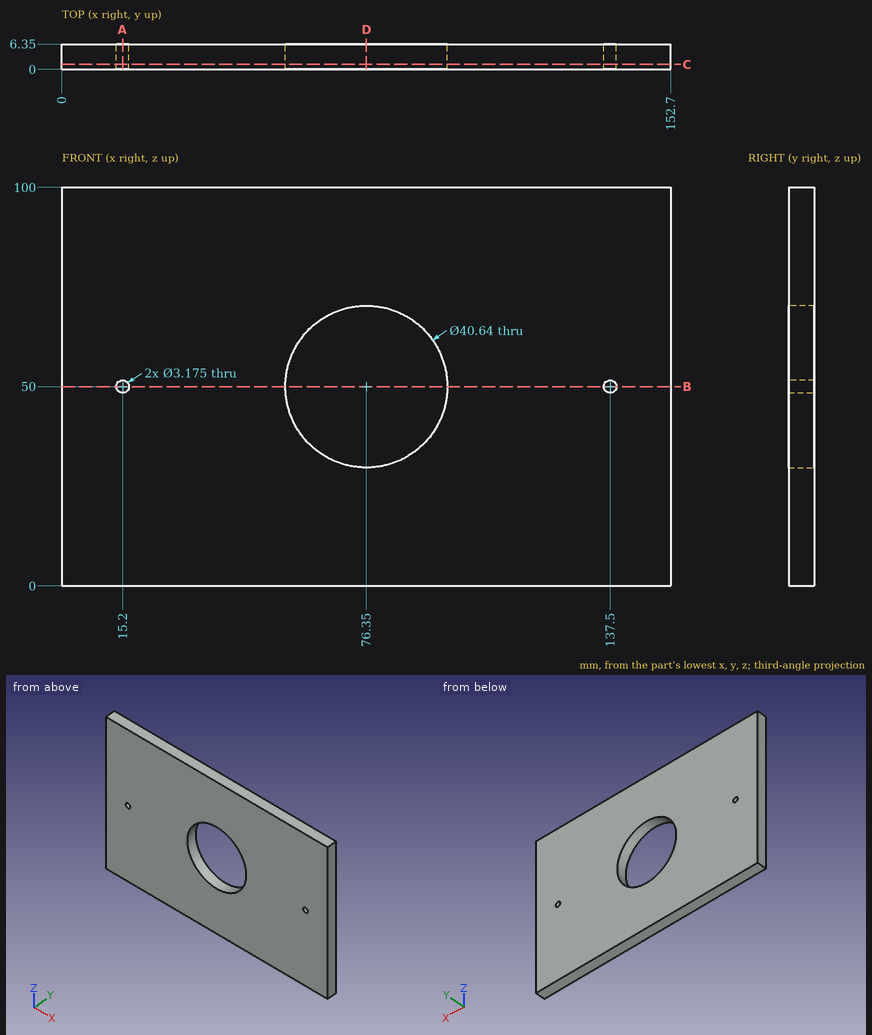
Design review of the part shown in the three views and the two pictorial views. Dimensions are in mm from the part's minimum x, y and z. Give positions to 0.01 mm unless a question says otherwise; leave off trailing zeros. Loops run counter-clockwise (first coordinate to the right, second up) from the corner with the lowest first, then second, coordinate; pieces in that order, holes last. Notation, with made-up numbers: (12, -29) - (69, -29) arc R29 ccw to (69, -4) - close; hole circle Ø3 at (86.5, -4). An arc over 180 degrees is marked (long way). Use CSV: the item, a comma, the result in double quotes. Start each with the question number.
1. Add section C-C (y = 1.25). Count the separate pieces of the cut face and the enclosed holes in it, plus the area to 3 significant figures.
2. Add section B-B (z = 50). State the section outline as (x, y) points.
3. Wall thickness on L1, parallel to X at y = 4, z = 50; L2, parallel to Z at x = 137.5, y = 4.75; L3, parallel to X at y = 2, z = 47: over which ranges is each line inside the solid? List them lowest first.
4. Add section D-D (x = 76.35). State the section outline as (y, z) points, plus the area to 3 significant figures.
5. Add section A-A (x = 15.2). State the section outline as (y, z) points, plus the area to 3 significant figures.
Results found:
1,separate pieces,"1"
1,enclosed holes,"3"
1,area,"14,000 mm²"
2,outline,"(0, 0) - (13.61, 0) - (13.61, 6.35) - (0, 6.35) - close; (16.79, 0) - (56.03, 0) - (56.03, 6.35) - (16.79, 6.35) - close; (96.67, 0) - (135.91, 0) - (135.91, 6.35) - (96.67, 6.35) - close; (139.09, 0) - (152.7, 0) - (152.7, 6.35) - (139.09, 6.35) - close"
3,L1,"x = 0 to 13.61, 16.79 to 56.03, 96.67 to 135.91, 139.09 to 152.7"
3,L2,"z = 0 to 48.41, 51.59 to 100"
3,L3,"x = 0 to 56.25, 96.45 to 152.7"
4,outline,"(0, 0) - (6.35, 0) - (6.35, 29.68) - (0, 29.68) - close; (0, 70.32) - (6.35, 70.32) - (6.35, 100) - (0, 100) - close"
4,area,"377 mm²"
5,outline,"(0, 0) - (6.35, 0) - (6.35, 48.41) - (0, 48.41) - close; (0, 51.59) - (6.35, 51.59) - (6.35, 100) - (0, 100) - close"
5,area,"615 mm²"
